from build123d import *

# Parameters (mm, degrees)
F2_DEPTH = 240


# Not quite as in the source:
# - ends of sketch curves that miss each other by under 0.0002 mm in the source are joined


with BuildPart() as f2:
    # F1 (on Front) → F2 (new body, symmetric)
    with BuildSketch(Plane.XZ):
        with BuildLine():
            Line((-8.250056, 12.999986), (-4.300056, 12.999986))
            ThreePointArc((-4.300056, 12.999986), (-4.0879239656, 13.0878539656), (-4.000056, 13.299986))
            Line((-4.000056, 13.299986), (-4.000056, 14.699986))
            ThreePointArc((-4.000056, 14.699986), (-4.0879239656, 14.9121180344), (-4.300056, 14.999986))
            Line((-4.300056, 14.999986), (-13.000056, 14.999986))
            ThreePointArc((-13.000056, 14.999986), (-14.4142695624, 14.4141995624), (-15.000056, 12.999986))
            Line((-15.000056, 12.999986), (-15.000056, 4.299986))
            ThreePointArc((-15.000056, 4.299986), (-14.9121880344, 4.0878539656), (-14.700056, 3.999986))
            Line((-14.700056, 3.999986), (-13.300056, 3.999986))
            ThreePointArc((-13.300056, 3.999986), (-13.0879239656, 4.0878539656), (-13.000056, 4.299986))
            Line((-13.000056, 4.299986), (-13.000056, 8.249986))
            Line((-13.000056, 8.249986), (-9.66427, 8.249986))
            Line((-9.66427, 8.249986), (-6.000056, 4.585772))
            Line((-6.000056, 4.585772), (-6.000056, 0.653576))
            ThreePointArc((-6.000056, 0.653576), (-5.9830189324, 0.5241665494), (-5.9330687764, 0.4035761291))
            Line((-5.9330687764, 0.4035761291), (-5.700056, -1.4e-05))
            Line((-5.700056, -1.4e-05), (-5.933069, -0.403604))
            ThreePointArc((-5.933069, -0.403604), (-6.000056, -0.653604), (-5.9330687764, -0.9036038709))
            Line((-5.9330687764, -0.9036038709), (-5.751033, -1.2189))
            Line((-5.751033, -1.2189), (-6.000056, -2.500014))
            Line((-6.000056, -2.500014), (-6.000056, -4.5858))
            Line((-6.000056, -4.5858), (-9.66427, -8.250014))
            Line((-9.66427, -8.250014), (-13.000056, -8.250014))
            Line((-13.000056, -8.250014), (-13.000056, -4.300014))
            ThreePointArc((-13.000056, -4.300014), (-13.0879239656, -4.0878819656), (-13.300056, -4.000014))
            Line((-13.300056, -4.000014), (-14.700056, -4.000014))
            ThreePointArc((-14.700056, -4.000014), (-14.9121880344, -4.0878819656), (-15.000056, -4.300014))
            Line((-15.000056, -4.300014), (-15.000056, -13.000014))
            ThreePointArc((-15.000056, -13.000014), (-14.4142695624, -14.4142275624), (-13.000056, -15.000014))
            Line((-13.000056, -15.000014), (12.999944, -15.000014))
            ThreePointArc((12.999944, -15.000014), (14.4141575624, -14.4142275624), (14.999944, -13.000014))
            Line((14.999944, -13.000014), (14.999944, 12.999986))
            ThreePointArc((14.999944, 12.999986), (14.4141575624, 14.4141995624), (12.999944, 14.999986))
            Line((12.999944, 14.999986), (4.299944, 14.999986))
            ThreePointArc((4.299944, 14.999986), (4.0878119656, 14.9121180344), (3.999944, 14.699986))
            Line((3.999944, 14.699986), (3.999944, 13.299986))
            ThreePointArc((3.999944, 13.299986), (4.0878119656, 13.0878539656), (4.299944, 12.999986))
            Line((4.299944, 12.999986), (8.249944, 12.999986))
            Line((8.249944, 12.999986), (8.249944, 9.6642))
            Line((8.249944, 9.6642), (4.58573, 5.999986))
            Line((4.58573, 5.999986), (0.653534, 5.999986))
            ThreePointArc((0.653534, 5.999986), (0.5241245494, 5.9829489324), (0.4035341291, 5.9329987764))
            Line((0.4035341291, 5.9329987764), (-5.6e-05, 5.699986))
            Line((-5.6e-05, 5.699986), (-0.403646, 5.932999))
            ThreePointArc((-0.403646, 5.932999), (-0.653646, 5.999986), (-0.9036458709, 5.9329987764))
            Line((-0.9036458709, 5.9329987764), (-1.218942, 5.750963))
            Line((-1.218942, 5.750963), (-2.500056, 5.999986))
            Line((-2.500056, 5.999986), (-4.585842, 5.999986))
            Line((-4.585842, 5.999986), (-8.250056, 9.6642))
            Line((-8.250056, 9.6642), (-8.250056, 12.999986))
        make_face()
        with BuildLine():
            ThreePointArc((-8.189375, -13.000014), (-8.339375082, -12.9598215738), (-8.4491827159, -12.8500138359))
            ThreePointArc((-8.4491827159, -12.8500138359), (-9.2743948384, -12.3508472042), (-10.1375690315, -12.7810479782))
            ThreePointArc((-10.1375690315, -12.7810479782), (-13.2041723505, -12.8608903949), (-12.3498940253, -9.9145979306))
            Line((-12.3498940253, -9.9145979306), (-11.07346, -9.450014))
            Line((-11.07346, -9.450014), (-8.450056, -9.450014))
            ThreePointArc((-8.450056, -9.450014), (-8.0673725676, -9.3738935325), (-7.7429492188, -9.1571207812))
            Line((-7.7429492188, -9.1571207812), (-4.878736, -6.292907))
            ThreePointArc((-4.878736, -6.292907), (-4.5543124324, -6.0761344675), (-4.171629, -6.000014))
            Line((-4.171629, -6.000014), (4.171517, -6.000014))
            ThreePointArc((4.171517, -6.000014), (4.5542004324, -6.0761344675), (4.8786237812, -6.2929072188))
            Line((4.8786237812, -6.2929072188), (7.957051, -9.371334))
            ThreePointArc((7.957051, -9.371334), (8.1738235325, -9.6957575676), (8.249944, -10.078441))
            Line((8.249944, -10.078441), (8.249944, -12.000014))
            ThreePointArc((8.249944, -12.000014), (7.9570507812, -12.7071207812), (7.249944, -13.000014))
            Line((7.249944, -13.000014), (-8.189375, -13.000014))
        make_face(mode=Mode.SUBTRACT)
        with BuildLine():
            ThreePointArc((9.5477956661, -11.3422641215), (9.8734155063, -9.8734855063), (11.3421941215, -9.5478656661))
            Line((11.3421941215, -9.5478656661), (12.349782, -9.914598))
            ThreePointArc((12.349782, -9.914598), (13.0434468843, -13.0435168843), (9.9145279306, -12.3498520253))
            Line((9.9145279306, -12.3498520253), (9.5477956661, -11.3422641215))
        make_face(mode=Mode.SUBTRACT)
        with BuildLine():
            ThreePointArc((-9.5479076661, 11.3422361215), (-9.8735275063, 9.8734575063), (-11.3423061215, 9.5478376661))
            Line((-11.3423061215, 9.5478376661), (-12.349894, 9.91457))
            ThreePointArc((-12.349894, 9.91457), (-13.0435588843, 13.0434888843), (-9.9146399306, 12.3498240253))
            Line((-9.9146399306, 12.3498240253), (-9.5479076661, 11.3422361215))
        make_face(mode=Mode.SUBTRACT)
        with BuildLine():
            ThreePointArc((3.2531309855, 0.9883049956), (3.399944, -1.4e-05), (3.2531309855, -0.9883329956))
            ThreePointArc((3.2531309855, -0.9883329956), (3.2974111593, -1.3177976431), (3.5754529349, -1.5000144258))
            ThreePointArc((3.5754529349, -1.5000144258), (3.8792555231, -1.6685151025), (3.999944, -1.99428))
            Line((3.999944, -1.99428), (3.999944, -3.500014))
            ThreePointArc((3.999944, -3.500014), (3.8534973906, -3.8535673906), (3.499944, -4.000014))
            Line((3.499944, -4.000014), (1.99421, -4.000014))
            ThreePointArc((1.99421, -4.000014), (1.6684451025, -3.8793255231), (1.4999444822, -3.5755229263))
            ThreePointArc((1.4999444822, -3.5755229263), (1.3177276431, -3.2974811593), (0.9882590481, -3.2532021585))
            ThreePointArc((0.9882590481, -3.2532021585), (-5.6e-05, -3.400014), (-0.9883749956, -3.2532009855))
            ThreePointArc((-0.9883749956, -3.2532009855), (-1.3178396431, -3.2974811593), (-1.5000564258, -3.5755229349))
            ThreePointArc((-1.5000564258, -3.5755229349), (-1.6685571025, -3.8793255231), (-1.994322, -4.000014))
            Line((-1.994322, -4.000014), (-3.500056, -4.000014))
            ThreePointArc((-3.500056, -4.000014), (-3.8536093906, -3.8535673906), (-4.000056, -3.500014))
            Line((-4.000056, -3.500014), (-4.000056, -1.99428))
            ThreePointArc((-4.000056, -1.99428), (-3.8793675231, -1.6685151025), (-3.5755649263, -1.5000144822))
            ThreePointArc((-3.5755649263, -1.5000144822), (-3.2975231593, -1.3177976431), (-3.2532441585, -0.9883290481))
            ThreePointArc((-3.2532441585, -0.9883290481), (-3.400056, -1.4e-05), (-3.2532429855, 0.9883049956))
            ThreePointArc((-3.2532429855, 0.9883049956), (-3.2975231593, 1.3177696431), (-3.5755649349, 1.4999864258))
            ThreePointArc((-3.5755649349, 1.4999864258), (-3.8793675231, 1.6684871025), (-4.000056, 1.994252))
            Line((-4.000056, 1.994252), (-4.000056, 3.499986))
            ThreePointArc((-4.000056, 3.499986), (-3.8536093906, 3.8535393906), (-3.500056, 3.999986))
            Line((-3.500056, 3.999986), (-1.994322, 3.999986))
            ThreePointArc((-1.994322, 3.999986), (-1.6685571025, 3.8792975231), (-1.5000564822, 3.5754949263))
            ThreePointArc((-1.5000564822, 3.5754949263), (-1.3178396431, 3.2974531593), (-0.9883710481, 3.2531741585))
            ThreePointArc((-0.9883710481, 3.2531741585), (-5.6e-05, 3.399986), (0.9882629956, 3.2531729855))
            ThreePointArc((0.9882629956, 3.2531729855), (1.3177276431, 3.2974531593), (1.4999444258, 3.5754949349))
            ThreePointArc((1.4999444258, 3.5754949349), (1.6684451025, 3.8792975231), (1.99421, 3.999986))
            Line((1.99421, 3.999986), (3.499944, 3.999986))
            ThreePointArc((3.499944, 3.999986), (3.8534973906, 3.8535393906), (3.999944, 3.499986))
            Line((3.999944, 3.499986), (3.999944, 1.994252))
            ThreePointArc((3.999944, 1.994252), (3.8792555231, 1.6684871025), (3.5754529263, 1.4999864822))
            ThreePointArc((3.5754529263, 1.4999864822), (3.2974111593, 1.3177696431), (3.2531309855, 0.9883049956))
        make_face(mode=Mode.SUBTRACT)
        with BuildLine():
            ThreePointArc((6.2928372188, -4.8786937812), (6.0760644675, -4.5542704324), (5.999944, -4.171587))
            Line((5.999944, -4.171587), (5.999944, 4.171559))
            ThreePointArc((5.999944, 4.171559), (6.0760644675, 4.5542424324), (6.2928372188, 4.8786657812))
            Line((6.2928372188, 4.8786657812), (9.157051, 7.742879))
            ThreePointArc((9.157051, 7.742879), (9.3738235325, 8.0673025676), (9.449944, 8.449986))
            Line((9.449944, 8.449986), (9.449944, 11.07339))
            Line((9.449944, 11.07339), (9.914528, 12.349824))
            ThreePointArc((9.914528, 12.349824), (12.8608203949, 13.2041023505), (12.7809779799, 10.1374990291))
            ThreePointArc((12.7809779799, 10.1374990291), (12.3507772042, 9.2743248384), (12.8499438252, 8.4491126972))
            ThreePointArc((12.8499438252, 8.4491126972), (12.9597515738, 8.339305082), (12.999944, 8.189305))
            Line((12.999944, 8.189305), (12.999944, -7.250014))
            ThreePointArc((12.999944, -7.250014), (12.7070507812, -7.9571207812), (11.999944, -8.250014))
            Line((11.999944, -8.250014), (10.078371, -8.250014))
            ThreePointArc((10.078371, -8.250014), (9.6956875676, -8.1738935325), (9.3712642188, -7.9571207812))
            Line((9.3712642188, -7.9571207812), (6.2928372188, -4.8786937812))
        make_face(mode=Mode.SUBTRACT)
    extrude(amount=F2_DEPTH, both=True)


solid = f2.part
Verification items for the finished model (mm, model axes). A direction names the side the tool comes from. Give positions to 0.01 mm unless a question says otherwise; leave off trailing zeros. Answer as a JSON object with one key per item and string values. Group by question number.
1) Scan lines: line 1 along Z through (x, y) = (1.25, -110.5); line 2 along X through (y, z) = (66.5, -4.5); line 3 along X through (y, z) = (57, 11.75). Record each from-to range of solid material in increasing order. Write a range as [from, to].
2) Access from +Z, -Z, +X, -X, +Y, -Y to the whole of each face (thin tool, end or side, straight path). Record for faces 5 (the face through (0, -3, -13)), 6 (the face through (0, 240, 4)).
3) Depth check by flat-ended pin: pin 1 Ø0.5 at (y, z) = (-97.5, 3) entering from -X; pin 2 Ø8 at (x, z) = (1.5, -11.5) entering from -Y; pin 3 Ø1.2 at (x, y) = (-3, 109.5) entering from +Z. Enter the tip coordinate at first touch or a pass-through.
4) Cross-section at A-A (y = 42). Give the number of separate pieces and of enclosed holes in the cut face, then the cut area to 3 significant figures.
5) Mould release check, pull along Z, two halves, no side actions. Record for faces 1 (the face through (-15, -3, -9)), 2 (the face through (13, -3, 1)), 3 (the face through (0, -3, -6)), 4 (the face through (-9, -3, 15)): released by +Z, released by -Z, zero draft, split by the parting line, or undercut.
Result sheet:
{
 "1": {"line 1": "z = [-15, -13], [-6, -3.26], [3.26, 6]", "line 2": "x = [-15, -13], [-6, 6.06], [13, 15]", "line 3": "x = [-15, -13.6], [-9.7, -8.25], [8.25, 9.7], [13.6, 15]"},
 "2": {"face 5": "+Y, -Y", "face 6": "+Z, -Z, +X, -X, +Y"},
 "3": {"pin 1": "stops at x = -6", "pin 2": "stops at y = -240", "pin 3": "stops at z = 6"},
 "4": {"separate pieces": "1", "enclosed holes": "5", "area": "339 mm2"},
 "5": {"face 1": "zero draft", "face 2": "undercut", "face 3": "undercut", "face 4": "released by +Z"}
}
